CAD build for the part. Positions are in the model's coordinates, mm. Face numbers are marked on the shaded views. A direction names the side the tool comes from. Coordinates: 2 decimals unless noted, no trailing zeros. Loops run counter-clockwise (first coordinate to the right, second up) from the corner with the lowest first, then second, coordinate; pieces in that order, holes last. Notation, with made-up numbers: (8, 19) - (25, 19) arc R15 ccw to (25, 42) - close; hole circle Ø7 at (9.5, 67.25). An arc over 180 degrees is marked (long way). Put each result on its own line as item: value.
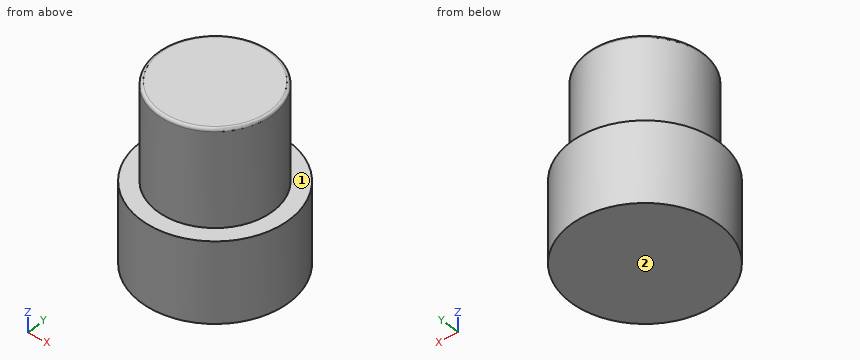
Autodesk Inventor part; units mm, degrees
ref_plane "YZ Plane" through (0, 0, 0) normal (1, 0, 0) x (0, 1, 0)
ref_plane "XZ Plane" through (0, 0, 0) normal (0, 1, 0) x (-1, 0, 0)
ref_plane "XY Plane" through (0, 0, 0) normal (0, 0, 1) x (1, 0, 0)
sketch "Sketch1" plane through (0, 0, 0) normal (0, 0, 1) x (1, 0, 0)
  circle A0 centre (0, 0) radius 3.9
  dimension "d0" = 7.8
extrude "Extrusion1" add sketch "Sketch1" along normal blind 12
sketch "Sketch2" plane through (0, 0, 0) normal (0, 0, -1) x (-1, 0, 0)
  circle A0 centre (0, 0) radius 5
  dimension "d3" = 10
extrude "Extrusion2" add sketch "Sketch2" against normal blind 5.45
fillet "Fillet1" radius 0.2 1 edges at (-3.9, 0, 12)
properties part number "ResetButton"
Q1. Slice it at C-C, the plane z = 7.25. Give the cut face in (x, y).
Determined:
outline: circle Ø7.8 at (0, 0)
Q2. Slice it at A-A, the plane x = 0. Give the cut face in (y, z), then the cut area to 3 significant figures.
Determined:
outline: (-5, 0) - (5, 0) - (5, 5.45) - (3.9, 5.45) - (3.9, 11.8) arc R0.2 ccw to (3.7, 12) - (-3.7, 12) arc R0.2 ccw to (-3.9, 11.8) - (-3.9, 5.45) - (-5, 5.45) - close
area: 106 mm2
Q3. Pin check, flat tips, straight feed: pin 1 Ø2 at (y, z) = (0.5, 10.5) entering from -X; pin 2 Ø2 at (y, z) = (3, 8.5) entering from -X; pin 3 Ø1.5 at (y, z) = (2.5, 9.5) entering from -X. Stop position of each tip, or through.
Determined:
pin 1: x = -3.9
pin 2: x = -3.35
pin 3: x = -3.49
Q4. Tool access for the marked faces 1 and 2: list every direction of +Z, -Z, +X, -X, +Y, -Y with a clear straight run to the whole face (end or side of a thin tool).
Determined:
face 1: +Z
face 2: -Z, +X, -X, +Y, -Y
Q5. Wall check: L1, parallel to Z at x = 3.25, y = 3.5; L2, parallel to X at y = 3, z = 7.5; L3, parallel to Y at x = -3, z = 4. Give the ranges that are in metal, low to high. Write a range as from..to.
Determined:
L1: 0..5.45
L2: -2.49..2.49
L3: -4..4
Q6. Slice it at D-D, the plane z = 4.75. Give the cut face in (x, y).
Determined:
outline: circle Ø10 at (0, 0)
